```python
from build123d import *

# Parameters (mm, degrees)
EXTRUDE_1_DEPTH        = 2040
SKETCH_2_R             = 8.75
CUT_EXTRUDE_1_DEPTH    = 14
CUT_EXTRUDE_2_REACH    = 2042.407
SKETCH_3_R             = 5.5
PATTERN_LINEAR_1_COUNT = 20
PATTERN_LINEAR_1_PITCH = 105


with BuildPart() as part:
    # 草图1 → 凸台-拉伸1 (new body)
    with BuildSketch(Plane(origin=(0, 0, 0), x_dir=(0, 0, -1), z_dir=(1, 0, 0))):
        with BuildLine():
            Line((-20.5, 0), (20.5, 0))
            Line((20.5, 0), (22.5, 2))
            Line((22.5, 2), (22.5, 18))
            Line((22.5, 18), (20.5, 20))
            Line((20.5, 20), (17.5, 20))
            Line((17.5, 20), (17.5, 24))
            Line((17.5, 24), (20.5, 24))
            Line((20.5, 24), (22.5, 26))
            Line((22.5, 26), (22.5, 32))
            ThreePointArc((22.5, 32), (21.914213562, 33.414213562), (20.5, 34))
            Line((20.5, 34), (-20.5, 34))
            ThreePointArc((-20.5, 34), (-21.914213562, 33.414213562), (-22.5, 32))
            Line((-22.5, 32), (-22.5, 26))
            Line((-22.5, 26), (-20.5, 24))
            Line((-20.5, 24), (-17.5, 24))
            Line((-17.5, 24), (-17.5, 20))
            Line((-17.5, 20), (-20.5, 20))
            Line((-20.5, 20), (-22.5, 18))
            Line((-22.5, 18), (-22.5, 2))
            Line((-22.5, 2), (-20.5, 0))
        make_face()
    extrude(amount=EXTRUDE_1_DEPTH)

    # 草图2 → 切除-拉伸1 (cut)
    with BuildSketch(Plane(origin=(0, 34, 0), x_dir=(1, 0, 0), z_dir=(0, 1, 0))):
        with Locations(Location((22.5, 0, 0), (0, 0, 270))):
            Circle(SKETCH_2_R)
    cut_extrude_1 = extrude(amount=-CUT_EXTRUDE_1_DEPTH, mode=Mode.SUBTRACT)

    # 草图3 → 切除-拉伸2 (cut, up to next)
    with BuildSketch(Plane.XZ, mode=Mode.PRIVATE) as cut_extrude_2_sk1:
        with Locations(Location((22.5, 0, 0), (0, 0, 270))):
            Circle(SKETCH_3_R)
    cut_extrude_2_tool1 = extrude(cut_extrude_2_sk1.sketch, amount=-CUT_EXTRUDE_2_REACH, mode=Mode.PRIVATE) & part.part
    cut_extrude_2 = cut_extrude_2_tool1.solids().sort_by_distance((22.5, 0, 0))[0]
    add(cut_extrude_2, mode=Mode.SUBTRACT)

    # 阵列(线性)1: 切除-拉伸1, 切除-拉伸2 ×20
    with Locations(*[(i * PATTERN_LINEAR_1_PITCH, 0, 0) for i in range(1, PATTERN_LINEAR_1_COUNT)]):
        add(cut_extrude_1, mode=Mode.SUBTRACT)
        add(cut_extrude_2, mode=Mode.SUBTRACT)


solid = part.part
```
Verification items for the finished model (mm, model axes). Give positions to 0.01 mm unless a question says otherwise; leave off trailing zeros. Write each loop counter-clockwise with the first axis right and the second up, starting at its lowest first coordinate (ties: lowest second). Pieces come first, ordered by that corner, then holes. Notation, with made-up numbers: (50.25, 84.5) - (88.25, 84.5) arc R34 cw to (88.25, 122.5) - close; hole circle Ø7 at (16.5, 34). An arc over 180 degrees is marked (long way). Put each result on its own line as item: value.
Q1. Depth check by flat-ended pin: P1, Ø10, axis at x = 652.5, z = 0, coming from the -Y side; P2, Ø20, axis at x = 1177.5, z = 0, coming from the +Y side; P3, Ø1.5, axis at x = 878, y = 20.5, coming from the +Z side. Enter the tip coordinate at first touch or a pass-through.
Result:
P1: through
P2: y = 34
P3: z = 20.75
Q2. Section check B-B on x = 1546. Record the cut outline in (y, z), and give its area (3 significant figures).
Result:
outline: (0, -20.5) - (2, -22.5) - (18, -22.5) - (20, -20.5) - (20, -17.5) - (24, -17.5) - (24, -20.5) - (26, -22.5) - (32, -22.5) arc R2 ccw to (34, -20.5) - (34, 20.5) arc R2 ccw to (32, 22.5) - (26, 22.5) - (24, 20.5) - (24, 17.5) - (20, 17.5) - (20, 20.5) - (18, 22.5) - (2, 22.5) - (0, 20.5) - close
area: 1,480 mm2
Q3. Scan lines: probe 1 along Z at (x, y) = (22, 15); probe 2 along Z at (x, y) = (1492.5, 31.25); probe 3 along Y at (x, z) = (1301, 20). Record each from-to range of solid material in increasing order. Write a range as from..to.
Result:
probe 1: -22.5..-5.48, 5.48..22.5
probe 2: -22.5..-8.75, 8.75..22.5
probe 3: 0..20, 24..34
Q4. Section check A-A on y = 10. Count the separate pieces of the cut face and the enclosed holes in it, and give its area (3 significant figures).
Result:
separate pieces: 1
enclosed holes: 20
area: 89,900 mm2
